For this review, use the dimensioned drawing (mm, ordinates from the lowest corner) and the shaded views. A direction names the side the tool comes from. Round coordinates to 2 decimals unless told otherwise and drop trailing zeros. Loops run counter-clockwise (first coordinate to the right, second up) from the corner with the lowest first, then second, coordinate; pieces in that order, holes last. Notation, with made-up numbers: M -37.5,-25.75 L 20.5,-25.75 A27 cw 20.5,1.25 Z; hole C 22.5,4 d9. An arc over 180 degrees is marked long. One line per item, written item: value. Start each with the question number.
Item 1: For the marked faces 1 and 2, list the 3-axis set-ups (+Z, -Z, +X, -X, +Y, -Y) from which the entire face can be reached by the end or side of a thin tool; tool diameter is ignored.
Item 2: We need section D-D (x = 11.5). Write out the cut boundary in (y, z).
Item 3: We need section A-A (z = 31). Write out the cut boundary in (x, y), then the cut area to 3 significant figures.
Item 4: We need section B-B (x = 49.5). Write out the cut boundary in (y, z), then the cut area to 3 significant figures.
Item 5: Mouldability with a two-part tool opening along X and no side actions: class the marked faces 3, 4, 5 and 6 as released by +X, released by -X, zero draft, split by the parting line, or undercut.
Item 6: Clearance check with a flat-ended pin moving along its axis: pin 1 (4 mm diameter, centred on x = 12, y = 28.5, fed in from +Z). State where the tip first meets the part, or that it passes through.
Item 7: For line 1 along Y through (x, z) = (15, 35); line 2 along X through (y, z) = (13, 9); line 3 along Z through (x, y) = (18, 36.5), list the stretches that pass through material, from the lowest coordinate up.
Item 8: We need section C-C (y = 66). Write out the cut boundary in (x, z), then the cut area to 3 significant figures.
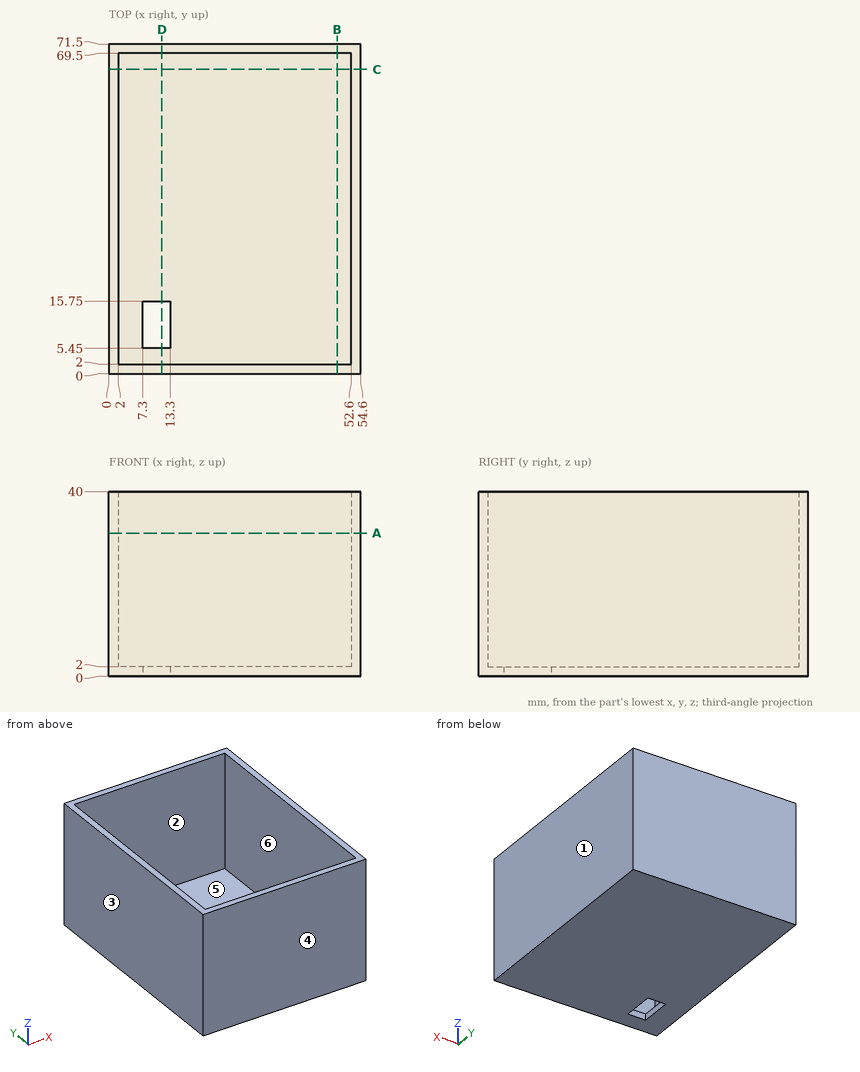
A:
1. face 1: +Z, -Z, +X, +Y, -Y
1. face 2: +Z
2. outline: M 0,0 L 5.45,0 L 5.45,2 L 2,2 L 2,40 L 0,40 Z; M 15.75,0 L 71.5,0 L 71.5,40 L 69.5,40 L 69.5,2 L 15.75,2 Z
3. outline: M 0,0 L 54.6,0 L 54.6,71.5 L 0,71.5 Z; hole M 2,2 L 52.6,2 L 52.6,69.5 L 2,69.5 Z
3. area: 488 mm2
4. outline: M 0,0 L 71.5,0 L 71.5,40 L 69.5,40 L 69.5,2 L 2,2 L 2,40 L 0,40 Z
4. area: 295 mm2
5. face 3: released by -X
5. face 4: zero draft
5. face 5: undercut
5. face 6: undercut
6. pin 1: z = 2
7. line 1: 0 to 2, 69.5 to 71.5
7. line 2: 0 to 2, 52.6 to 54.6
7. line 3: 0 to 2
8. outline: M 0,0 L 54.6,0 L 54.6,40 L 52.6,40 L 52.6,2 L 2,2 L 2,40 L 0,40 Z
8. area: 261 mm2
